```python
from build123d import *

# Parameters (mm, degrees)
SKETCH_1_W             = 2490
SKETCH_1_H             = 48
EXTRUDE_1_DEPTH        = 25
SKETCH_2_W             = 115
SKETCH_2_H             = 6
CUT_EXTRUDE_1_DEPTH    = 7.5
DRAFT_1_ANGLE          = 45
MIRROR_START           = 13
MIRROR_1_DEPTH         = 6
PATTERN_START          = 13
PATTERN_LINEAR_1_DEPTH = 6
CUT_EXTRUDE_2_REACH    = 2492.588


# Read off the part's stored shape, not the designer's step: 镜向1, 阵列(线性)1
with BuildPart() as part:
    # 草图1 → 凸台-拉伸1 (new body)
    with BuildSketch(Plane.XY):
        with Locations((1245, 0)):
            Rectangle(SKETCH_1_W, SKETCH_1_H)
    extrude(amount=EXTRUDE_1_DEPTH)

    # 草图2 → 切除-拉伸1 (cut)
    with BuildSketch(Plane(origin=(0, 24, 0), x_dir=(1, 0, 0), z_dir=(0, 1, 0))):
        with Locations((1900, -16)):
            Rectangle(SKETCH_2_W, SKETCH_2_H)
    extrude(amount=-CUT_EXTRUDE_1_DEPTH, mode=Mode.SUBTRACT)

    # 拔模1
    draft_1_faces = [part.faces().sort_by_distance(p)[0] for p in [
        (1957.5, 20.25, 16),
        (1842.5, 20.25, 16),
    ]]
    draft(draft_1_faces, Plane(origin=(0, 16.5, 0), x_dir=(1, 0, 0), z_dir=(0, 1, 0)), DRAFT_1_ANGLE)

    # 镜向1 outline → 镜向1 (cut)
    with BuildSketch(Plane.XY.offset(MIRROR_START)):
        Polygon((1957.5, -16.5), (1842.5, -16.5), (1835, -24), (1965, -24), align=None)
    extrude(amount=MIRROR_1_DEPTH, mode=Mode.SUBTRACT)

    # 阵列(线性)1 outline → 阵列(线性)1 (cut)
    with BuildSketch(Plane.XY.offset(PATTERN_START)):
        Polygon((215, -24), (207.5, -16.5), (92.5, -16.5), (85, -24), align=None)
        Polygon((207.5, 16.5), (215, 24), (85, 24), (92.5, 16.5), align=None)
    extrude(amount=PATTERN_LINEAR_1_DEPTH, mode=Mode.SUBTRACT)

    # 草图3 → 切除-拉伸2 (cut, up to next)
    with BuildSketch(Plane.XZ.offset(24), mode=Mode.PRIVATE) as cut_extrude_2_sk1:
        Polygon((2400, 0), (2490, 0), (2490, 15), align=None)
    cut_extrude_2_tool1 = extrude(cut_extrude_2_sk1.sketch, amount=-CUT_EXTRUDE_2_REACH, mode=Mode.PRIVATE) & part.part
    add(cut_extrude_2_tool1.solids().sort_by_distance((2460, -24, 5))[0], mode=Mode.SUBTRACT)


solid = part.part
```
Design review of the part built by this model. Coordinates are the model's own, in mm. Give positions to 0.01 mm unless a question says otherwise; leave off trailing zeros. Order: outer loops, then holes, each group sorted by start corner. A loop starts at its lowest first (then second) coordinate and runs counter-clockwise, first axis right, second up. Notation, with made-up numbers: (-36, 67) -> (13, 67) arc R25 cw to (13, 90) -> close; hole circle Ø10 at (21.5, 5). An arc over 180 degrees is marked (long way). Write each question's results on one line, items separated by ' | '. Start each with the question number.
Q1. Add section B-B on z = 7.75. Give the boundary of the cut face in (x, y), and give its area (3 significant figures).
Q2. Mouldability with a two-part tool opening along X and no side actions: class faces 1 (the flat face through (2445.6, -0.3, 7.6)), 2 (the flat face through (1228, 0, 25)) as +X half, -X half, draft (parallel to the pull), parting line (faces both ways), or undercut.
Q3. Add section A-A on x = 173. Give the boundary of the cut face in (y, z).
Q4. For pin 1 (1.8 mm diameter, centred on x = 158, z = 14.5, fed in from -Y), flat-tipped, find the tip position at first contact; note if it passes through.
Q5. Wall thickness on L1, parallel to Z at x = 1947, y = -20; L2, parallel to Y at x = 1890.5, z = 16.75: over which ranges is each line inside the solid? List them lowest first. Write a range as from..to.
Found:
1) outline: (0, -24) -> (2446.5, -24) -> (2446.5, 24) -> (0, 24) -> close | area: 117,000 mm2
2) face 1: +X half | face 2: draft
3) outline: (-24, 0) -> (24, 0) -> (24, 13) -> (16.5, 13) -> (16.5, 19) -> (24, 19) -> (24, 25) -> (-24, 25) -> (-24, 19) -> (-16.5, 19) -> (-16.5, 13) -> (-24, 13) -> close
4) pin 1: stops at y = -16.5
5) L1: z = 0..13, 19..25 | L2: y = -16.5..16.5
